For this review, take the finished solid that the model builds, in its own axes (mm). A direction names the side the tool comes from. Coordinates: 2 decimals unless noted, no trailing zeros. Loops run counter-clockwise (first coordinate to the right, second up) from the corner with the lowest first, then second, coordinate; pieces in that order, holes last. Notation, with made-up numbers: M -14.75,-1.75 L -10.75,-1.75 A27 cw -10.75,27.25 Z; hole C 86,-15 d3. An arc over 180 degrees is marked long. Put each result on its own line as item: value.
```python
from build123d import *

# Parameters (mm, degrees)
EXTRUDE_1_DEPTH          = 45
SKETCH_3_R               = 8
EXTRUDE_2_DEPTH          = 10
FILLET_1_RADIUS          = 22.5
FILLET_1_LENGTH          = 10.659867141
CUT_EXTRUDE_1_DEPTH      = 97.311280041
CUT_EXTRUDE_1_DEPTH_BACK = 97.311280041


with BuildPart() as part:
    # 草图2 → 凸台-拉伸1 (new body)
    with BuildSketch(Plane.XY):
        Polygon((0, 0), (60, 0), (60, 12), (-1.661115121, 12), (-5.903755809, 7.757359313), (-6.61086259, 8.464466094), (-51.860645565, -36.785316881), (-44.322981223, -44.322981223), align=None)
    extrude(amount=EXTRUDE_1_DEPTH)

    # 草图3 → 凸台-拉伸2 (add)
    with BuildSketch(Plane(origin=(0, 0, 0), x_dir=(-1, 0, 0), z_dir=(0, 0, -1))):
        with BuildLine():
            Line((-60, 12), (-26.595595968, 51.809818513))
            ThreePointArc((-26.595595968, 51.809818513), (-8.866562585, 56.560298691), (1.661115121, 41.525216758))
            Line((1.661115121, 41.525216758), (1.661115121, 12))
            Line((1.661115121, 12), (-60, 12))
        make_face()
        with Locations((-14.338884879, 41.525216758)):
            Circle(SKETCH_3_R, mode=Mode.SUBTRACT)
    extrude(amount=-EXTRUDE_2_DEPTH)

    # 圆角1: full round fillet: the end face becomes a half cylinder, R = half its width
    fillet_1_face = Plane((-48.091813394, -40.554149052, 22.5), x_dir=(-0.707106781187, 0.707106781187, 0), z_dir=(-0.707106781187, -0.707106781187, 0))  # on the end face: x along it, z out of the body
    fillet_1_slab = fillet_1_face.offset(-FILLET_1_RADIUS / 2) * Box(FILLET_1_LENGTH, 2 * FILLET_1_RADIUS, FILLET_1_RADIUS, mode=Mode.PRIVATE)  # the body's end, R deep
    fillet_1_round = Plane((-32.181910817, -24.644246475, 22.5), x_dir=(-0.707106781187, -0.707106781187, 0), z_dir=(-0.707106781187, 0.707106781187, 0)) * Cylinder(FILLET_1_RADIUS, FILLET_1_LENGTH, mode=Mode.PRIVATE)  # its axis R under the face
    add(fillet_1_slab - fillet_1_round, mode=Mode.SUBTRACT)

    # 草图6 → 切除-拉伸1 (cut, two sides: drawn at the far end of the back side and taken through both)
    with BuildSketch(Plane(origin=(-7.537664342, 7.537664342, 0), x_dir=(0, 0, 1), z_dir=(-0.7071067811865487, 0.7071067811865465, 0)).offset(-CUT_EXTRUDE_1_DEPTH_BACK)):
        with BuildLine():
            Line((30.5, -20.182161171), (30.5, -40.182161171))
            ThreePointArc((30.5, -40.182161171), (22.5, -48.182161171), (14.5, -40.182161171))
            Line((14.5, -40.182161171), (14.5, -20.182161171))
            ThreePointArc((14.5, -20.182161171), (22.5, -12.182161171), (30.5, -20.182161171))
        make_face()
    extrude(amount=CUT_EXTRUDE_1_DEPTH + CUT_EXTRUDE_1_DEPTH_BACK, mode=Mode.SUBTRACT)


solid = part.part
```
(1) Add section C-C (z = 6). Write out the cut boundary in (x, y), plus the area to 3 significant figures.
Determined:
outline: M -46.77,-31.69 L -39.23,-39.23 L 0,0 L 60,0 L 60,12 L 26.6,51.81 A16 ccw -1.66,41.53 L -1.66,12 L -5.9,7.76 L -6.61,8.46 Z; hole C 14.34,41.53 d16
area: 3,030 mm^2
(2) Draft analysis for pull direction Y (two halves, no side actions). For faces 5 (the flat face through (-1.661, 27, 5)), 6 (the cylindrical face through (9.12, 56.65, 4.93)), 7 (the cylindrical face through (16.073, 33.715, 4.93)), state which applies: +Y half, -Y half, draft (parallel to the pull), parting line (faces both ways), or undercut.
Determined:
face 5: draft
face 6: +Y half
face 7: undercut
(3) Tool access review of faces 1 (the flat face through (-25, -18, 14.5)), 2 (the cylindrical face through (-48.14, -40.5, 22.01)), 3 (the flat face through (22, 30, 10)), 4 (the flat face through (30, 0, 22)): name each direction out of +Z, -Z, +X, -X, +Y, -Y from which nothing blocks a thin tool from reaching the whole face with its end or side.
Determined:
face 1: none
face 2: -X, -Y
face 3: +Z, +X, -X, +Y
face 4: +Z, -Z, +X, -Y
(4) Add section D-D (x = 3). Write out the cut boundary in (y, z), plus the area to 3 significant figures.
Determined:
outline: M 0,0 L 52.81,0 L 52.81,10 L 12,10 L 12,45 L 0,45 Z
area: 948 mm^2
(5) For pin 1 (11 mm diameter, centred on y = 21.5, z = 4.5, fed in from -X); pin 2 (8 mm diameter, centred on y = -1, z = 34.5, fed in from +X); pin 3 (2 mm diameter, centred on x = -19, z = 38, fed in from -Y); pin 4 (8 mm diameter, centred on x = 24.5, z = 39, fed in from +Y), all flat-tipped, find the tip position at first contact; note any pin that passes through.
Determined:
pin 1: stops at x = -1.66
pin 2: stops at x = 60
pin 3: stops at y = -20
pin 4: stops at y = 12
(6) Add section A-A (y = -18.5). Write out the cut boundary in (x, z), plus the area to 3 significant figures.
Determined:
outline: M -33.58,0 L -18.5,0 L -18.5,14.5 L -33.58,14.5 Z; M -33.58,30.5 L -18.5,30.5 L -18.5,45 L -33.58,45 Z
area: 437 mm^2
(7) Add section B-B (z = 21). Write out the cut boundary in (x, y), plus the area to 3 significant figures.
Determined:
outline: M -51.83,-36.75 L -44.29,-44.29 L -33.97,-33.97 L -41.51,-26.43 Z; M -16.25,-1.18 L -8.71,-8.71 L 0,0 L 60,0 L 60,12 L -1.66,12 L -5.9,7.76 L -6.61,8.46 Z
area: 1,050 mm^2
(8) Wall thickness on line 1 along Y through (x, z) = (50, 35); line 2 along X through (y, z) = (38.5, 7); line 3 along Z through (x, y) = (46, 28.5): over which ranges is each line inside the solid? List them lowest first. Write a range as [from, to].
Determined:
line 1: y = [0, 12]
line 2: x = [-1.66, 6.93], [21.74, 37.76]
line 3: z = [0, 10]
